For this review, take the finished solid that the model builds, in its own axes (mm). A direction names the side the tool comes from. Give positions to 0.01 mm unless a question says otherwise; leave off trailing zeros. Order: outer loops, then holes, each group sorted by start corner. A loop starts at its lowest first (then second) coordinate and runs counter-clockwise, first axis right, second up. Notation, with made-up numbers: (-34.5, -24.5) - (-30.5, -24.5) arc R19 cw to (-30.5, 12.5) - close; hole circle Ø11 at (3, 32.25). An arc over 180 degrees is marked (long way). Answer as a JSON object with one key per item and string values. Group by question number.
Autodesk Inventor part; units mm, degrees
ref_plane "YZ Plane" through (0, 0, 0) normal (1, 0, 0) x (0, 1, 0)
ref_plane "XZ Plane" through (0, 0, 0) normal (0, 1, 0) x (-1, 0, 0)
ref_plane "XY Plane" through (0, 0, 0) normal (0, 0, 1) x (1, 0, 0)
sketch "Sketch1" plane through (0, 0, 0) normal (0, 0, 1) x (1, 0, 0)
  circle A0 centre (31.75, 28.575) radius 3.3782
  circle A1 centre (31.75, 9.525) radius 3.3782
  circle A2 centre (31.75, -9.525) radius 3.3782
  circle A3 centre (31.75, -28.575) radius 3.3782
  circle A4 centre (67.1293, 62.0712) radius 6.35 construction
  circle A5 centre (67.1293, -62.0713) radius 6.35 construction
  line L0 (19.05, 74.7712) -> (19.05, -74.7713)
  line L1 (19.05, -74.7713) -> (67.1293, -74.7713)
  line L2 (67.1293, -74.7713) -> (67.1293, -68.4213)
  line L3 (19.05, 74.7712) -> (67.1293, 74.7712)
  line L4 (67.1293, 74.7712) -> (67.1293, 68.4212)
  line L5 (67.1293, 62.0712) -> (67.1293, 55.7212) construction
  line L6 (67.1293, -55.7213) -> (67.1293, -62.0713) construction
  line L7 (44.45, 44.45) -> (44.45, -44.45)
  line L8 (44.45, -44.45) -> (67.1293, -55.7213)
  line L9 (44.45, 44.45) -> (67.1293, 55.7212)
  arc A6 (67.1293, 68.4212) -> (67.1293, 55.7212) centre (67.1293, 62.0712) ccw
  line L10 (67.1293, 68.4212) -> (67.1293, 62.0712) construction
  arc A7 (67.1293, -55.7213) -> (67.1293, -68.4213) centre (67.1293, -62.0713) ccw
  line L11 (67.1293, -62.0713) -> (67.1293, -68.4213) construction
  point P0 (0, 0)
  dimension "d0" = 88.9
  dimension "d2" = 12.7
  dimension "d3" = 12.7
  dimension "d4" = 12.7
  dimension "d5" = 12.7
extrude "Extrusion1" add sketch "Sketch1" along normal blind 1.5875
fillet "Fillet1" radius 6.35 4 edges at (67.1293, 74.7712, 0.7937) (67.1293, -74.7713, 0.7937) (19.05, -74.7713, 0.7937) (19.05, 74.7712, 0.7937)
equation "\"d4\" = d3"
equation "\"d5\" = d2"
properties part number "V5 Shooter Guide Rail Support Plate" material "Aluminum-6061"
1) Consider section B-B (z = 0.25). Give the number of separate pieces and of enclosed holes in the cut face, plus the area to 3 significant figures.
2) For line 1 (Y direction, x = 31.75, z = 0.45); line 2 (Y direction, x = 30, z = 0.35); line 3 (Y direction, x = 54, z = 1.05), list the stretches that pass through material, from the lowest coordinate up.
3) For pin 1 (8 mm diameter, centred on x = 31.75, y = -28.575, fed in from +Z); pin 2 (0.5 mm diameter, centred on y = 10, z = 1, fed in from +X), all flat-tipped, find the tip position at first contact; note any pin that passes through.
4) For faces 1 (the face through (37, 1, 0)), 2 (the face through (55.631, 50.007, 0.783)), list the 3-axis set-ups (+Z, -Z, +X, -X, +Y, -Y) from which the entire face can be reached by the end or side of a thin tool; tool diameter is ignored.
5) Consider section C-C (x = 64). Give the boundary of the cut face in (y, z).
6) Consider section D-D (x = 55.5). Give the boundary of the cut face in (y, z).
7) Mouldability with a two-part tool opening along Y and no side actions: class faces 3 (the face through (21, -73, 1)), 4 (the face through (65.32, 72.86, 0.8)), 5 (the face through (55.631, -50.007, 0.783)) as released by +Y, released by -Y, zero draft, split by the parting line, or undercut.
8) Consider section A-A (x = 31.75). Give the boundary of the cut face in (y, z).
Result set:
{
 "1": {"separate pieces": "1", "enclosed holes": "4", "area": "4,610 mm2"},
 "2": {"line 1": "y = -74.77 to -31.95, -25.2 to -12.9, -6.15 to 6.15, 12.9 to 25.2, 31.95 to 74.77", "line 2": "y = -74.77 to -31.46, -25.69 to -12.41, -6.64 to 6.64, 12.41 to 25.69, 31.46 to 74.77", "line 3": "y = -74.77 to -49.2, 49.2 to 74.77"},
 "3": {"pin 1": "stops at z = 1.59", "pin 2": "stops at x = 44.45"},
 "4": {"face 1": "-Z, +X, -X, +Y, -Y", "face 2": "+Z, -Z, +X"},
 "5": {"outline": "(-73.89, 0) - (-67.6, 0) - (-67.6, 1.59) - (-73.89, 1.59) - close; (-56.55, 0) - (-54.17, 0) - (-54.17, 1.59) - (-56.55, 1.59) - close; (54.17, 0) - (56.55, 0) - (56.55, 1.59) - (54.17, 1.59) - close; (67.6, 0) - (73.89, 0) - (73.89, 1.59) - (67.6, 1.59) - close"},
 "6": {"outline": "(-74.77, 0) - (-49.94, 0) - (-49.94, 1.59) - (-74.77, 1.59) - close; (49.94, 0) - (74.77, 0) - (74.77, 1.59) - (49.94, 1.59) - close"},
 "7": {"face 3": "released by -Y", "face 4": "released by +Y", "face 5": "undercut"},
 "8": {"outline": "(-74.77, 0) - (-31.95, 0) - (-31.95, 1.59) - (-74.77, 1.59) - close; (-25.2, 0) - (-12.9, 0) - (-12.9, 1.59) - (-25.2, 1.59) - close; (-6.15, 0) - (6.15, 0) - (6.15, 1.59) - (-6.15, 1.59) - close; (12.9, 0) - (25.2, 0) - (25.2, 1.59) - (12.9, 1.59) - close; (31.95, 0) - (74.77, 0) - (74.77, 1.59) - (31.95, 1.59) - close"}
}
